Source: CAD feature listing. Evaluate the final solid. Frame: model axes, mm. Coordinates: 2 decimals unless noted, no trailing zeros. Order: outer loops, then holes, each group sorted by start corner. A loop starts at its lowest first (then second) coordinate and runs counter-clockwise, first axis right, second up.
```python
from build123d import *

# Parameters (mm, degrees)
SKETCH_1_W      = 57
SKETCH_1_H      = 55
SKETCH_1_R      = 1.6
SKETCH_1_W_2    = 30
SKETCH_1_H_2    = 4
EXTRUDE_1_DEPTH = 2
FILLET_1_R      = 2


with BuildPart() as part:
    # 草图1 → 凸台-拉伸1 (new body)
    with BuildSketch(Plane.XY):
        Rectangle(SKETCH_1_W, SKETCH_1_H)
        with Locations((24.75, 23.7)):
            Circle(SKETCH_1_R, mode=Mode.SUBTRACT)
        with Locations(Location((-24.75, 23.7, 0), (0, 0, 180))):
            Circle(SKETCH_1_R, mode=Mode.SUBTRACT)
        with Locations(Location((24.75, -23.7, 0), (0, 0, 180))):
            Circle(SKETCH_1_R, mode=Mode.SUBTRACT)
        with Locations((-24.75, -23.7)):
            Circle(SKETCH_1_R, mode=Mode.SUBTRACT)
        with Locations((0, 17.5)):
            Circle(SKETCH_1_R, mode=Mode.SUBTRACT)
        with Locations((0, -17.5)):
            Circle(SKETCH_1_R, mode=Mode.SUBTRACT)
        Polygon((-2.880312196, 0), (-23.5, 19.896189986), (-23.5, -19.896189986), align=None, mode=Mode.SUBTRACT)
        Polygon((0, -2.77924861), (-12.146960531, -14.5), (0, -14.5), (12.146960531, -14.5), align=None, mode=Mode.SUBTRACT)
        with Locations((0, 22.5)):
            Rectangle(SKETCH_1_W_2, SKETCH_1_H_2, mode=Mode.SUBTRACT)
        Polygon((2.880312196, 0), (23.5, 19.896189986), (23.5, -19.896189986), align=None, mode=Mode.SUBTRACT)
        Polygon((0, 2.77924861), (12.146960531, 14.5), (0, 14.5), (-12.146960531, 14.5), align=None, mode=Mode.SUBTRACT)
        with Locations((0, -22.5)):
            Rectangle(SKETCH_1_W_2, SKETCH_1_H_2, mode=Mode.SUBTRACT)
    extrude(amount=EXTRUDE_1_DEPTH)

    # 圆角1
    fillet_1_edges = [part.edges().sort_by_distance(p)[0] for p in [
        (23.5, 19.896189986, 1),
        (2.880312196, 0, 1),
        (23.5, -19.896189986, 1),
        (-15, 24.5, 1),
        (-15, 20.5, 1),
        (15, 20.5, 1),
        (15, 24.5, 1),
        (12.146960531, -14.5, 1),
        (0, -2.77924861, 1),
        (-23.5, 19.896189986, 1),
        (-23.5, -19.896189986, 1),
        (-2.880312196, 0, 1),
        (-12.146960531, -14.5, 1),
        (-28.5, -27.5, 1),
        (-28.5, 27.5, 1),
        (28.5, 27.5, 1),
        (28.5, -27.5, 1),
        (12.146960531, 14.5, 1),
        (0, 2.77924861, 1),
        (-12.146960531, 14.5, 1),
        (15, -24.5, 1),
        (15, -20.5, 1),
        (-15, -24.5, 1),
        (-15, -20.5, 1),
    ]]
    fillet(fillet_1_edges, radius=FILLET_1_R - 0.0001)  # a hair under: the kernel refuses the full size


solid = part.part
```
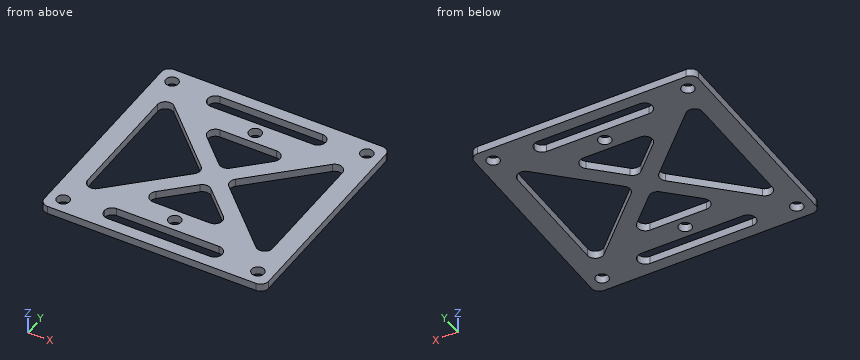
1. Section query B-B, the plane y = -23.7. Output: boundary loops of the cut face in (x, z).
2. Contact query for a flat-ended pin moving along its axis: P1, Ø3, axis at x = -24.75, y = -23.7, coming from the +Z side. Output: stop coordinate, or through.
3. Section query D-D, the plane x = -11.5. Output: boundary loops of the cut face in (y, z), plus the area to 3 significant figures.
4. Material intervals for line 1 along Y through (x, z) = (24.75, 1.55); line 2 along Y through (x, z) = (11.5, 1); line 3 along Y through (x, z) = (-13, 1.55), sorted ascending.
5. Section query A-A, the plane x = -24.75. Output: boundary loops of the cut face in (y, z), plus the area to 3 significant figures.
6. Section query C-C, the plane x = 0. Output: boundary loops of the cut face in (y, z), plus the area to 3 significant figures.
Answer key:
1. outline: (-28.5, 0) - (-26.35, 0) - (-26.35, 2) - (-28.5, 2) - close; (-23.15, 0) - (-14.6, 0) - (-14.6, 2) - (-23.15, 2) - close; (14.6, 0) - (23.15, 0) - (23.15, 2) - (14.6, 2) - close; (26.35, 0) - (28.5, 0) - (28.5, 2) - (26.35, 2) - close
2. P1: passes through
3. outline: (-27.5, 0) - (-24.5, 0) - (-24.5, 2) - (-27.5, 2) - close; (-20.5, 0) - (-8.32, 0) - (-8.32, 2) - (-20.5, 2) - close; (8.32, 0) - (20.5, 0) - (20.5, 2) - (8.32, 2) - close; (24.5, 0) - (27.5, 0) - (27.5, 2) - (24.5, 2) - close
3. area: 60.7 mm2
4. line 1: y = -27.5 to -25.3, -22.1 to 22.1, 25.3 to 27.5
4. line 2: y = -27.5 to -24.5, -20.5 to -8.32, 8.32 to 20.5, 24.5 to 27.5
4. line 3: y = -27.5 to -24.5, -20.5 to -9.76, 9.76 to 20.5, 24.5 to 27.5
5. outline: (-27.5, 0) - (-25.3, 0) - (-25.3, 2) - (-27.5, 2) - close; (-22.1, 0) - (22.1, 0) - (22.1, 2) - (-22.1, 2) - close; (25.3, 0) - (27.5, 0) - (27.5, 2) - (25.3, 2) - close
5. area: 97.2 mm2
6. outline: (-27.5, 0) - (-24.5, 0) - (-24.5, 2) - (-27.5, 2) - close; (-20.5, 0) - (-19.1, 0) - (-19.1, 2) - (-20.5, 2) - close; (-15.9, 0) - (-14.5, 0) - (-14.5, 2) - (-15.9, 2) - close; (-3.56, 0) - (3.56, 0) - (3.56, 2) - (-3.56, 2) - close; (14.5, 0) - (15.9, 0) - (15.9, 2) - (14.5, 2) - close; (19.1, 0) - (20.5, 0) - (20.5, 2) - (19.1, 2) - close; (24.5, 0) - (27.5, 0) - (27.5, 2) - (24.5, 2) - close
6. area: 37.4 mm2
